Check sheet for the modelled part. Datum: model origin and axes. Units: mm. Face numbers are marked on the shaded views. A direction names the side the tool comes from. Give positions to 0.01 mm unless a question says otherwise; leave off trailing zeros. Loops run counter-clockwise (first coordinate to the right, second up) from the corner with the lowest first, then second, coordinate; pieces in that order, holes last. Notation, with made-up numbers: (5.25, 68) -> (55.25, 68) arc R20 cw to (55.25, 96) -> close; hole circle Ø1 at (40.25, 59). An arc over 180 degrees is marked (long way). Write each question's results on one line, items separated by ' | '. Start each with the question number.
Item 1: Access from +Z, -Z, +X, -X, +Y, -Y to the whole of each face (thin tool, end or side, straight path). Record for the marked faces 1, 2 and 3.
Item 2: Cross-section at A-A on x = 19.25. Enter the section's corners in (y, z).
Item 3: Cross-section at C-C on y = 24.9. Enter the section's corners in (x, z).
Item 4: Cross-section at D-D on x = 13.5. Enter the section's corners in (y, z).
Item 5: Scan lines: line 1 along X through (y, z) = (24.9, 15.15); line 2 along X through (y, z) = (37, 2.75); line 3 along X through (y, z) = (31, 4.5). Record each from-to range of solid material in increasing order.
Item 6: Cross-section at B-B on y = 15. Enter the section's corners in (x, z), then the cut area to 3 significant figures.
Item 7: Mould release check, pull along X, two halves, no side actions. Record for the marked faces 4, 5 and 6: pulls with the +X half, pulls with the -X half, needs draft (parallel to the pull), parting line crosses it, or undercut.
Item 8: Gauge pin test, flat ends, axial feed: pin 1 Ø1 at (x, y) = (23.5, 33) entering from +Z; pin 2 Ø1.5 at (x, y) = (11.5, 33) entering from +Z; pin 3 Ø1.6 at (x, z) = (27.5, 0.5) entering from -Y; pin 4 Ø1.2 at (x, y) = (5.5, 26) entering from -Z. Record the tip position at first contact, or that the pin passes through.
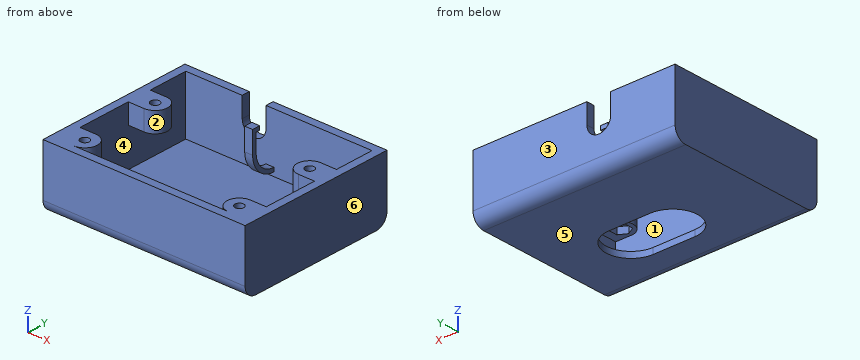
Autodesk Inventor part; units mm, degrees
ref_plane "Work Plane1" through (0, 0, 16) normal (0, 0, 1) x (1, 0, 0)
ref_plane "Work Plane2" through (22.25, 40, 4.75) normal (0, 0, 1) x (1, 0, 0)
ref_plane "Work Plane4" through (22.25, 40, 11) normal (-1, 0, 0) x (0, 0, 1)
sketch "Sketch1" plane through (0, 0, 0) normal (0, 0, 1) x (1, 0, 0)
  line L0 (0, 0) -> (51, 0)
  line L1 (51, 0) -> (51, 40)
  line L2 (51, 40) -> (0, 40)
  line L3 (0, 40) -> (0, 0)
  dimension "d0" = 40
  dimension "d1" = 51
extrude "Extrusion1" add sketch "Sketch1" along normal blind 16
sketch "Sketch2" plane through (0, 0, 16) normal (0, 0, 1) x (1, 0, 0)
  line L0 (2, 38) -> (49, 38)
  line L1 (49, 38) -> (49, 2)
  line L2 (49, 2) -> (2, 2)
  line L3 (2, 2) -> (2, 38)
  line L4 (51, 40) -> (0, 40)
  line L5 (0, 40) -> (0, 0)
  line L6 (51, 0) -> (51, 40)
  line L7 (0, 0) -> (51, 0)
  dimension "d4" = 2
  dimension "d5" = 2
  dimension "d6" = 2
  dimension "d7" = 2
extrude "Extrusion2" cut sketch "Sketch2" against normal blind 14.5 contours L0 L1 L2 L3
fillet "Fillet1" radius 3 2 edges at (25.5, 40, 0) (25.5, 0, 0)
sketch "Sketch3" plane through (0, 0, 0) normal (0, 0, -1) x (-1, 0, 0)
  line L0 (-51, 3) -> (-51, 37)
  line L1 (0, 37) -> (0, 3)
  line L2 (-51, 37) -> (0, 37)
  line L3 (0, 3) -> (-51, 3)
  circle A0 centre (-33.5, 15) radius 6.25
  circle A1 centre (-23, 15) radius 6.25
  line L4 (-33.5, 21.25) -> (-23, 21.25)
  line L5 (-33.5, 8.75) -> (-23, 8.75)
  line L6 (0, 40) -> (-51, 40)
  point P0 (0, 0)
  point P1 (-28.25, 21.25)
  dimension "d49" = 12.5
  dimension "d51" = 10.5
  dimension "d52" = 12.5
  dimension "d54" = 17.5
  dimension "d55" = 22.75
  dimension "d58" = 25
extrude "Extrusion3" cut sketch "Sketch3" against normal blind 14 contours A0 A1 | L4 A1 A0 | A0 A1 L5 | A1 A0 | A0 A1
sketch "Sketch4" plane through (0, 40, 16) normal (0, 1, 0) x (1, 0, 0)
  line L0 (35.25, 0) -> (21.25, 0)
  line L1 (21.25, 0) -> (21.25, 8)
  line L2 (21.25, 8) -> (35.25, 8)
  line L3 (35.25, 8) -> (35.25, 0)
  line L4 (51, 0) -> (0, 0)
  line L5 (0, 13) -> (0, 0)
  line L6 (51, 13) -> (51, 0)
  point P0 (0, 16)
  dimension "d18" = 14
  dimension "d19" = 8
  dimension "d20" = 21.25
  dimension "d21" = 15.75
ref_plane "Work Plane1" through (0, 0, 16) normal (0, 0, 1) x (1, 0, 0)
sketch "Sketch5" plane through (0, 0, 16) normal (0, 0, 1) x (1, 0, 0)
  circle A0 centre (6, 24.9) radius 3.1
  line L0 (49, 38) -> (49, 2)
  line L1 (6, 28) -> (2, 28)
  line L2 (6, 21.8) -> (2, 21.8)
  circle A1 centre (6, 24.9) radius 1.1
  line L3 (2, 2) -> (2, 38)
  line L4 (25.5, 34) -> (25.5, 3) construction
  line L5 (0, 3) -> (51, 3) construction
  line L6 (2, 2) -> (2, 38) construction
  line L7 (49, 38) -> (49, 2) construction
  circle A2 centre (6, 5.1) radius 3.1
  line L8 (6, 2) -> (2, 2)
  line L9 (6, 8.2) -> (2, 8.2)
  circle A3 centre (6, 5.1) radius 1.1
  line L10 (2, 38) -> (2, 2)
  line L11 (2, 38) -> (2, 2) construction
  circle A4 centre (45, 24.9) radius 3.1
  line L12 (45, 28) -> (49, 28)
  line L13 (45, 21.8) -> (49, 21.8)
  circle A5 centre (45, 24.9) radius 1.1
  line L14 (49, 2) -> (49, 38)
  line L15 (51, 3) -> (0, 3) construction
  line L16 (49, 2) -> (49, 38) construction
  line L17 (49, 38) -> (49, 2)
  line L18 (49, 38) -> (49, 2) construction
  line L19 (45, 8.2) -> (49, 8.2)
  circle A6 centre (45, 5.1) radius 3.1
  line L20 (45, 2) -> (49, 2)
  circle A7 centre (45, 5.1) radius 1.1
  line L21 (2, 38) -> (49, 38)
  line L22 (49, 2) -> (2, 2)
  point P0 (0, 0)
  point P1 (4, 28)
  point P2 (4, 2)
  point P3 (47, 28)
  point P4 (47, 2)
  point P5 (49, 8.2)
  point P6 (2, 2)
  point P7 (2, 8.2)
  point P8 (25.5, 38)
  dimension "d28" = 6.2
  dimension "d30" = 4
  dimension "d31" = 2.2
  dimension "d61" = 19.8
  dimension "d62" = 6.2
extrude "Extrusion5" add sketch "Sketch5" against normal blind 5 contours A0 | A0 L2 L3 L1 | L9 A2 L8 L3 | A2 | L0 L13 A4 L12 | A4 | A6 | A6 L19 L0 L20
sketch "Sketch6" plane through (0, 0, 11) normal (0, 0, -1) x (-1, 0, 0)
  circle A0 centre (-45, 24.9) radius 1.1
  line L0 (-45, 22.5906) -> (-47, 23.7453)
  line L1 (-47, 23.7453) -> (-47, 26.0547)
  line L2 (-47, 26.0547) -> (-45, 27.2094)
  line L3 (-45, 27.2094) -> (-43, 26.0547)
  line L4 (-43, 26.0547) -> (-43, 23.7453)
  line L5 (-43, 23.7453) -> (-45, 22.5906)
  arc A1 (-6, 28) -> (-6, 21.8) centre (-6, 24.9) ccw
  line L6 (-6, 22.5906) -> (-8, 23.7453)
  line L7 (-8, 23.7453) -> (-8, 26.0547)
  line L8 (-8, 26.0547) -> (-6, 27.2094)
  line L9 (-6, 27.2094) -> (-4, 26.0547)
  line L10 (-4, 26.0547) -> (-4, 23.7453)
  line L11 (-4, 23.7453) -> (-6, 22.5906)
  circle A2 centre (-6, 5.1) radius 1.1
  line L12 (-6, 2.7906) -> (-8, 3.9453)
  line L13 (-8, 3.9453) -> (-8, 6.2547)
  line L14 (-8, 6.2547) -> (-6, 7.4094)
  line L15 (-6, 7.4094) -> (-4, 6.2547)
  line L16 (-4, 6.2547) -> (-4, 3.9453)
  line L17 (-4, 3.9453) -> (-6, 2.7906)
  arc A3 (-45, 2) -> (-45, 8.2) centre (-45, 5.1) ccw
  line L18 (-45, 2.7906) -> (-47, 3.9453)
  line L19 (-47, 3.9453) -> (-47, 6.2547)
  line L20 (-47, 6.2547) -> (-45, 7.4094)
  line L21 (-45, 7.4094) -> (-43, 6.2547)
  line L22 (-43, 6.2547) -> (-43, 3.9453)
  line L23 (-43, 3.9453) -> (-45, 2.7906)
  circle A4 centre (-45, 5.1) radius 1.1
  circle A5 centre (-6, 24.9) radius 1.1
  point P0 (0, 0)
  point P1 (-6, 38)
  point P2 (-6, 5.1)
  point P3 (-45, 5.1)
  dimension "d45" = 4
extrude "Extrusion6" cut sketch "Sketch6" against normal blind 1.7
ref_plane "Work Plane2" through (22.25, 40, 4.75) normal (0, 0, 1) x (1, 0, 0)
sketch "Sketch10" plane through (0, 40, 16) normal (0, 1, 0) x (1, 0, 0)
  line L0 (45, 0) -> (6, 0)
  line L1 (16.25, 0) -> (22.25, 0)
  line L2 (22.25, 0) -> (22.25, 5)
  line L3 (22.25, 5) -> (16.25, 5)
  line L4 (16.25, 5) -> (16.25, 0)
  circle A0 centre (19.25, 5) radius 3
  line L5 (0, 13) -> (0, 0)
  point P0 (0, 16)
  point P1 (16.25, 5)
  point P2 (22.25, 0)
  dimension "d65" = 16.25
  dimension "d66" = 6
  dimension "d67" = 5
extrude "Extrusion9" cut sketch "Sketch10" against normal blind 2
ref_plane "Work Plane4" through (22.25, 40, 11) normal (-1, 0, 0) x (0, 0, 1)
sketch "Sketch12" plane through (22.25, 40, 11) normal (-1, 0, 0) x (0, 0, 1)
  line L0 (5, -2) -> (-9.5, -2)
  line L1 (-2.5, -7) -> (3, -7)
  line L2 (3, -7) -> (3, -8)
  arc A0 (-8.5, -2) -> (-2.5, -8) centre (-2.5, -2) ccw
  line L3 (3, -8) -> (-2.5, -8)
  arc A1 (-7.5, -2) -> (-2.5, -7) centre (-2.5, -2) ccw
  line L4 (3, -7) -> (2, -7)
  line L5 (2, -7) -> (2, -6)
  line L6 (2, -6) -> (3, -6)
  line L7 (3, -6) -> (3, -7)
  point P0 (-11, -40)
  point P1 (-3, -2)
  point P2 (3.5, -2)
  point P3 (2, -7)
  dimension "d73" = 1
  dimension "d74" = 5
  dimension "d77" = 1
  dimension "d78" = 1
  dimension "d79" = 1
  dimension "d80" = 4.5
  dimension "d81" = 5
extrude "Extrusion10" add sketch "Sketch12" against normal blind 2
properties part number "lidarhouse"
Answer sheet:
1) face 1: none | face 2: +Z | face 3: +Z, -Z, +X, -X, +Y
2) outline: (0, 3) arc R3 ccw to (3, 0) -> (10, 0) -> (10, 1.5) -> (2, 1.5) -> (2, 16) -> (0, 16) -> close; (20, 0) -> (37, 0) arc R3 ccw to (40, 3) -> (40, 8) -> (38, 8) -> (38, 1.5) -> (20, 1.5) -> close
3) outline: (0, 0) -> (51, 0) -> (51, 16) -> (46.1, 16) -> (46.1, 12.7) -> (47, 12.7) -> (47, 11) -> (49, 11) -> (49, 1.5) -> (2, 1.5) -> (2, 11) -> (4, 11) -> (4, 12.7) -> (4.9, 12.7) -> (4.9, 16) -> (0, 16) -> close; (7.1, 12.7) -> (8, 12.7) -> (8, 11) -> (9.1, 11) -> (9.1, 16) -> (7.1, 16) -> close; (41.9, 11) -> (43, 11) -> (43, 12.7) -> (43.9, 12.7) -> (43.9, 16) -> (41.9, 16) -> close
4) outline: (0, 3) arc R3 ccw to (3, 0) -> (37, 0) arc R3 ccw to (40, 3) -> (40, 16) -> (38, 16) -> (38, 1.5) -> (2, 1.5) -> (2, 16) -> (0, 16) -> close
5) line 1: x = 0 to 4.9, 7.1 to 9.1, 41.9 to 43.9, 46.1 to 51 | line 2: x = 0 to 2, 22.25 to 24.25, 49 to 51 | line 3: x = 0 to 2, 49 to 51
6) outline: (0, 0) -> (16.75, 0) -> (16.75, 1.5) -> (2, 1.5) -> (2, 16) -> (0, 16) -> close; (39.75, 0) -> (51, 0) -> (51, 16) -> (49, 16) -> (49, 1.5) -> (39.75, 1.5) -> close | area: 100 mm²
7) face 4: undercut | face 5: needs draft | face 6: pulls with the +X half
8) pin 1: stops at z = 14 | pin 2: stops at z = 1.5 | pin 3: stops at y = 0.53 | pin 4: stops at z = 0
